For this review, take the finished solid that the model builds, in its own axes (mm). Face numbers are marked on the shaded views. Give positions to 0.01 mm unless a question says otherwise; leave off trailing zeros. Order: outer loops, then holes, each group sorted by start corner. A loop starts at its lowest first (then second) coordinate and runs counter-clockwise, first axis right, second up. Notation, with made-up numbers: (35.5, 2) - (53.5, 2) arc R22 cw to (53.5, 38) - close; hole circle Ø9 at (17, 66.5). An arc over 180 degrees is marked (long way). One line per item, written item: value.
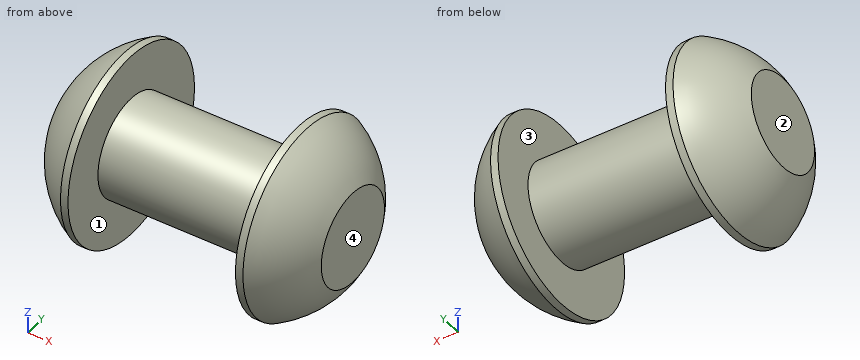
```python
from build123d import *


with BuildPart() as part:
    # Sketch2 → Revolve1 (revolve)
    with BuildSketch(Plane.XY):
        with BuildLine():
            ThreePointArc((0, 2.375), (0.992680215, 3.754414901), (2.37, 4.75))
            Line((2.37, 4.75), (2.75, 4.75))
            Line((2.75, 4.75), (2.75, 2.5))
            Line((2.75, 2.5), (11.25, 2.5))
            Line((11.25, 2.5), (11.25, 4.75))
            Line((11.25, 4.75), (11.63, 4.75))
            ThreePointArc((11.63, 4.75), (13.007319785, 3.754414901), (14, 2.375))
            Line((14, 2.375), (14, 0))
            Line((14, 0), (0, 0))
            Line((0, 0), (0, 2.375))
        make_face()
    revolve(axis=Axis((-1.178114582, 0, 0), (1, 0, 0)))


solid = part.part
```
(1) For P1, Ø1.5, axis at y = 3.5, z = 2, coming from the +X side; P2, Ø2, axis at x = 2.5, y = -2.5, coming from the -Z side; P3, Ø1.5, axis at x = 5.5, z = -0.5, coming from the +Y side, all flat-tipped, find the tip position at first contact; note any pin that passes through.
Answers below:
P1: stops at x = 13.43
P2: stops at z = -4.51
P3: stops at y = 2.5
(2) Take a section at C-C (x = 5). Write out the cut boundary in (y, z).
Answers below:
outline: circle Ø5 at (0, 0)
(3) Take a section at A-A (y = 0). Write out the cut boundary in (x, z) (3 decimals), then the cut area to 3 significant figures.
Answers below:
outline: (0, -2.375) arc R5.315 ccw to (2.37, -4.75) - (2.75, -4.75) - (2.75, -2.5) - (11.25, -2.5) - (11.25, -4.75) - (11.63, -4.75) arc R5.315 ccw to (14, -2.375) - (14, 2.375) arc R5.315 ccw to (11.63, 4.75) - (11.25, 4.75) - (11.25, 2.5) - (2.75, 2.5) - (2.75, 4.75) - (2.37, 4.75) arc R5.315 ccw to (0, 2.375) - close
area: 85.9 mm^2
(4) Draft analysis for pull direction X (two halves, no side actions). For the marked faces 1, 2, 3 and 4, state which applies: pulls with the +X half, pulls with the -X half, needs draft (parallel to the pull), parting line crosses it, or undercut.
Answers below:
face 1: undercut
face 2: pulls with the -X half
face 3: undercut
face 4: pulls with the +X half
(5) Wall thickness on line 1 (X direction, y = -1.75, z = -2.5); line 2 (X direction, y = -3.5, z = 1.5); line 3 (Y direction, x = 9.5, z = 1.75): over which ranges is each line inside the solid? List them lowest first. Write a range as from..to.
Answers below:
line 1: x = 0.4..2.75, 11.25..13.6
line 2: x = 1.05..2.75, 11.25..12.95
line 3: y = -1.79..1.79
